```python
from build123d import *

# Parameters (mm, degrees)
F0_W     = 40
F0_H     = 100
F0_R     = 17.5
F0_R_2   = 1.45
F1_DEPTH = 5
F2_W     = 5
F2_H     = 100
F3_DEPTH = 10
F4_R     = 17.5
F4_R_2   = 16.5
F5_DEPTH = 1


with BuildPart() as f1:
    # F0 (on Top) → F1 (new body)
    with BuildSketch(Plane.XY):
        Rectangle(F0_W, F0_H)
        with Locations((0.5, -26.2)):
            Circle(F0_R, mode=Mode.SUBTRACT)
        with Locations((0.5, -26.2)):
            Circle(F0_R)
        with Locations((0.5, -26.2)):
            Circle(F0_R_2, mode=Mode.SUBTRACT)
    extrude(amount=-F1_DEPTH)

    # F2 (on face) → F3 (join)
    with BuildSketch(Plane.XY):
        with Locations((-22.5, 0)):
            Rectangle(F2_W, F2_H)
        Polygon((-25, 50), (-20, 50), (20, 50), (20, 55), (-25, 55), align=None)
    extrude(amount=-F3_DEPTH)

    # F4 (on face) → F5 (cut)
    with BuildSketch(Plane.XY):
        with Locations((0.5, -26.2)):
            Circle(F4_R)
        with Locations((0.5, -26.2)):
            Circle(F4_R_2, mode=Mode.SUBTRACT)
    extrude(amount=-F5_DEPTH, mode=Mode.SUBTRACT)


solid = f1.part
```
Model file for the job. Use its own axes, mm. A direction names the side the tool comes from. Give positions to 0.01 mm unless a question says otherwise; leave off trailing zeros. Write each loop counter-clockwise with the first axis right and the second up, starting at its lowest first coordinate (ties: lowest second). Pieces come first, ordered by that corner, then holes. Notation, with made-up numbers: M -34,69 L -5,69 A10 cw -5,76 Z; hole C 58,66 d11. An arc over 180 degrees is marked long. Use a Markdown table: item, result.
1) Drill centre lines: line 1 (Y direction, x = 0.5, z = -0.3); line 2 (Y direction, x = 0.5, z = -3.7); line 3 (Y direction, x = 18, z = -8.5). Where is each one in solid material? Low to high. Write a range as from..to.
Responses:
| item | result |
|---|---|
| line 1 | y = -50..-43.7, -42.7..-27.65, -24.75..-9.7, -8.7..55 |
| line 2 | y = -50..-27.65, -24.75..55 |
| line 3 | y = 50..55 |
2) Pin check, flat tips, straight feed: pin 1 (5.5 mm diameter, centred on x = -8.5, z = -8, fed in from -Y); pin 2 (2.5 mm diameter, centred on y = -24, z = -8, fed in from +X); pin 3 (4 mm diameter, centred on x = 0.5, y = -26.2, fed in from -Z). Stop position of each tip, or through.
Responses:
| item | result |
|---|---|
| pin 1 | stops at y = 50 |
| pin 2 | stops at x = -20 |
| pin 3 | stops at z = -5 |
3) Pull direction X, two halves, no side cores. Call faces 1 (the flat face through (4, -26, 0)), 2 (the flat face through (-11, -14, -1)), 3 (the flat face through (20, 2, -3)), 4 (the cylindrical face through (16.238, -21.244, -0.493)): +X half, -X half, draft (parallel to the pull), parting line (faces both ways), or undercut.
Responses:
| item | result |
|---|---|
| face 1 | draft |
| face 2 | undercut |
| face 3 | +X half |
| face 4 | undercut |
4) Cut at C-C (y = 20.5). List the corners of the cut face in (x, z).
Responses:
| item | result |
|---|---|
| outline | M -25,-10 L -20,-10 L -20,-5 L 20,-5 L 20,0 L -25,0 Z |
5) Tool access for faces 5 (the cylindrical face through (0.186, -27.616, -2.465)), 6 (the cylindrical face through (-3.294, -43.284, -0.493)), 7 (the flat face through (-20, -1, -7)): list every direction of +Z, -Z, +X, -X, +Y, -Y with a clear straight run to the whole face (end or side of a thin tool).
Responses:
| item | result |
|---|---|
| face 5 | +Z, -Z |
| face 6 | +Z |
| face 7 | -Z, +X, -Y |
6) Cut at D-D (x = 13.5). List the corners of the cut face in (y, z), and give its area (3 significant figures).
Responses:
| item | result |
|---|---|
| outline | M -50,-5 L 50,-5 L 50,-10 L 55,-10 L 55,0 L -14.48,0 L -14.48,-1 L -16.04,-1 L -16.04,0 L -36.36,0 L -36.36,-1 L -37.92,-1 L -37.92,0 L -50,0 Z |
| area | 547 mm2 |
7) Cut at B-B (x = 0.5). List the corners of the cut face in (y, z).
Responses:
| item | result |
|---|---|
| outline | M -50,-5 L -27.65,-5 L -27.65,0 L -42.7,0 L -42.7,-1 L -43.7,-1 L -43.7,0 L -50,0 Z; M -24.75,-5 L 50,-5 L 50,-10 L 55,-10 L 55,0 L -8.7,0 L -8.7,-1 L -9.7,-1 L -9.7,0 L -24.75,0 Z |
8) Cut at A-A (y = -26.2). List the corners of the cut face in (x, z).
Responses:
| item | result |
|---|---|
| outline | M -25,-10 L -20,-10 L -20,-5 L -0.95,-5 L -0.95,0 L -16,0 L -16,-1 L -17,-1 L -17,0 L -25,0 Z; M 1.95,-5 L 20,-5 L 20,0 L 18,0 L 18,-1 L 17,-1 L 17,0 L 1.95,0 Z |
